Could you check a few things on this model? Use its own coordinates, in mm. A direction names the side the tool comes from. Coordinates: 2 decimals unless noted, no trailing zeros. Write each loop counter-clockwise with the first axis right and the second up, starting at its lowest first coordinate (ties: lowest second). Pieces come first, ordered by that corner, then holes. Notation, with made-up numbers: (6, 4) - (63, 4) arc R18 ccw to (63, 21) - close; hole circle Ø11 at (43, 28.5). An arc over 180 degrees is marked (long way). Answer as a JSON object with one key per item and string values. Group by question number.
1) If we section it at D-D (x = -3): Write out the boundary of the cut face in (y, z) (3 decimals).
2) Please list where these lines run through material, in increasing order: line 1 along X through (y, z) = (76.2, 55.25) (1 decimal); line 2 along X through (y, z) = (76, 54); line 3 along Y through (x, z) = (0, 3.75) (1 decimal).
3) We'd pull the mould along Z, two halves only. Please class faces 4 (the flat face through (0, -76, 49.276)), 5 (the flat face through (0, 1, 0)), 6 (the flat face through (-15.24, -16, 28)): released by +Z, released by -Z, zero draft, split by the parting line, or undercut.
4) If we section it at A-A (y = -66): Write out the boundary of the cut face in (x, z).
5) On a 3-axis mill with a long thin cutter (end or side, diameter ignored), from which of +Z, -Z, +X, -X, +Y, -Y can I reach the whole of each face in a straight line? I mean faces 1 (the flat face through (0, -59.69, 29)), 2 (the flat face through (0, 25.4, 29)), 3 (the flat face through (0, 76, 3.175)). Say none if no direction works.
6) Will these pins go through, and if not, where does the flat tip stop? pin 1 Ø9 at (x, z) = (-5.5, 25) entering from -Y; pin 2 Ø9 at (x, z) = (4, 23) entering from +Y.
7) If we section it at B-B (z = 16): Write out the boundary of the cut face in (x, y).
8) If we section it at C-C (x = 13.5): Write out the boundary of the cut face in (y, z).
```python
from build123d import *

# Parameters (mm, degrees)
BOSS_EXTRUDE1_DEPTH = 57.15
SKETCH2_W           = 44.45
SKETCH2_H           = 66.04
CUT_EXTRUDE1_DEPTH  = 57.15
SKETCH6_R           = 4.7625
CUT_EXTRUDE3_DEPTH  = 3.175
SKETCH8_R           = 0.79375
CUT_EXTRUDE4_DEPTH  = 58.15
SKETCH9_W           = 41.402
SKETCH9_H           = 31.75
CUT_EXTRUDE5_DEPTH  = 31.48


with BuildPart() as part:
    # Sketch1 → Boss-Extrude1 (new body)
    with BuildSketch(Plane.XY):
        with BuildLine():
            Line((-15.24, 76.2), (-15.24, -76.2))
            ThreePointArc((-15.24, -76.2), (0, -91.44), (15.24, -76.2))
            Line((15.24, -76.2), (15.24, 76.2))
            ThreePointArc((15.24, 76.2), (0, 91.44), (-15.24, 76.2))
        make_face()
    extrude(amount=BOSS_EXTRUDE1_DEPTH)

    # Sketch2 → Cut-Extrude1 (cut)
    with BuildSketch(Plane(origin=(15.24, 0, 0), x_dir=(0, 0, -1), z_dir=(1, 0, 0))):
        with Locations((-28.575, 58.42)):
            Rectangle(SKETCH2_W, SKETCH2_H)
    extrude(amount=-CUT_EXTRUDE1_DEPTH, mode=Mode.SUBTRACT)

    # Sketch6 → Cut-Extrude3 (cut)
    with BuildSketch(Plane.XY.offset(6.35)):
        with Locations((0, 76.2)):
            Circle(SKETCH6_R)
    extrude(amount=-CUT_EXTRUDE3_DEPTH, mode=Mode.SUBTRACT)

    # Sketch8 → Cut-Extrude4 (cut, through all)
    with BuildSketch(Plane(origin=(0, 0, 0), x_dir=(-1, 0, 0), z_dir=(0, 0, -1))):
        with Locations((0, 65.88125)):
            Circle(SKETCH8_R)
        with Locations((-10.31875, 76.2)):
            Circle(SKETCH8_R)
        with Locations((0, 86.51875)):
            Circle(SKETCH8_R)
        with Locations((10.31875, 76.2)):
            Circle(SKETCH8_R)
    extrude(amount=-CUT_EXTRUDE4_DEPTH, mode=Mode.SUBTRACT)

    # Sketch9 → Cut-Extrude5 (cut, through all)
    with BuildSketch(Plane(origin=(15.24, 0, 0), x_dir=(0, 0, -1), z_dir=(1, 0, 0))):
        with Locations((-28.575, -75.565)):
            Rectangle(SKETCH9_W, SKETCH9_H)
    extrude(amount=-CUT_EXTRUDE5_DEPTH, mode=Mode.SUBTRACT)


solid = part.part
```
Here are the results:
{
 "1": {"outline": "(-91.142, 0) - (91.142, 0) - (91.142, 6.35) - (79.899, 6.35) - (79.899, 3.175) - (72.501, 3.175) - (72.501, 6.35) - (25.4, 6.35) - (25.4, 50.8) - (91.142, 50.8) - (91.142, 57.15) - (-91.142, 57.15) - (-91.142, 49.276) - (-59.69, 49.276) - (-59.69, 7.874) - (-91.142, 7.874) - close"},
 "2": {"line 1": "x = -15.2 to -11.1, -9.5 to 9.5, 11.1 to 15.2", "line 2": "x = -15.24 to -11.09, -9.55 to 9.55, 11.09 to 15.24", "line 3": "y = -91.4 to 65.1, 66.7 to 71.4, 81 to 85.7, 87.3 to 91.4"},
 "3": {"face 4": "undercut", "face 5": "released by -Z", "face 6": "zero draft"},
 "4": {"outline": "(-15.24, 0) - (15.24, 0) - (15.24, 7.87) - (-15.24, 7.87) - close; (-15.24, 49.28) - (15.24, 49.28) - (15.24, 57.15) - (-15.24, 57.15) - close"},
 "5": {"face 1": "+X, -X, -Y", "face 2": "+X, -X, +Y", "face 3": "none"},
 "6": {"pin 1": "stops at y = -59.69", "pin 2": "stops at y = 25.4"},
 "7": {"outline": "(-15.24, -59.69) - (15.24, -59.69) - (15.24, 25.4) - (-15.24, 25.4) - close"},
 "8": {"outline": "(-83.27, 0) - (83.27, 0) - (83.27, 6.35) - (25.4, 6.35) - (25.4, 50.8) - (83.27, 50.8) - (83.27, 57.15) - (-83.27, 57.15) - (-83.27, 49.28) - (-59.69, 49.28) - (-59.69, 7.87) - (-83.27, 7.87) - close"}
}
